Autodesk Inventor part; units mm, degrees
ref_plane "YZ Plane" through (0, 0, 0) normal (1, 0, 0) x (0, 1, 0)
ref_plane "XZ Plane" through (0, 0, 0) normal (0, 1, 0) x (-1, 0, 0)
ref_plane "XY Plane" through (0, 0, 0) normal (0, 0, 1) x (1, 0, 0)
sketch "Esboço1" plane through (0, 0, 0) normal (0, 0, 1) x (1, 0, 0)
  line L0 (0, 0) -> (-70, 0)
  line L1 (0, 0) -> (0, 30)
  line L2 (-70, 30) -> (-70, 28)
  line L3 (-70, 28) -> (-18, 28)
  line L4 (-18, 28) -> (-58.0179, 28)
  line L5 (-18, 28) -> (-18, 25)
  line L6 (-18, 25) -> (-6, 25)
  line L7 (-6, 25) -> (-6, 0)
  line L8 (0, 30) -> (-6, 30)
  line L9 (-6, 30) -> (-6, 27.5)
  line L10 (-6, 27.5) -> (-9, 27.5)
  line L11 (-9, 27.5) -> (-9, 30)
  line L12 (-9, 30) -> (-12, 30)
  line L13 (-12, 30) -> (-12, 27.5)
  line L14 (-12, 27.5) -> (-15, 27.5)
  line L15 (-15, 27.5) -> (-15, 30)
  line L16 (-15, 30) -> (-70, 30)
  line L17 (-6, 0) -> (0, 0)
  dimension "d1" = 60
  dimension "d2" = 70
  dimension "d4" = 70
  dimension "d5" = 56
  dimension "d8" = 52
  dimension "d9" = 64
  dimension "d10" = 50
  dimension "d11" = 6
  dimension "d12" = 55
  dimension "d13" = 3
  dimension "d14" = 3
  dimension "d15" = 3
  dimension "d16" = 55
  dimension "d17" = 55
  dimension "d18" = 60
revolve "Revolução1" add sketch "Esboço1" angle 360 about axis through (0, 0, 0) along (-1, 0, 0)
chamfer "Chanfro1" distance 2 angle 45 1 edges at (0, -30, 0)
fillet "Arredondamento1" radius 2 1 edges at (-18, -28, 0)
sketch "Esboço2" plane through (0, 0, 0) normal (0, 0, 1) x (1, 0, 0)
  line L0 (-70, 0) -> (-40, 0)
  line L1 (-70, 0) -> (-90, 0)
  circle A0 centre (-90, 0) radius 32.5
  point P0 (0, 0)
  dimension "d24" = 70
  dimension "d25" = 30
  dimension "d26" = 20
  dimension "d27" = 65
  dimension "d28" = 90
extrude "Extrusão1" cut sketch "Esboço2" along normal mid plane 200000
sketch "Esboço3" plane through (0, 0, 0) normal (0, 1, 0) x (-1, 0, 0)
  line L0 (70, -15.6125) -> (70, 15.6125)
  line L1 (70, 0) -> (40, 0)
  line L2 (70, -15.6125) -> (70, 15.6125)
  circle A0 centre (40, 0) radius 12.5
  point P0 (0, 0)
  dimension "d32" = 30
  dimension "d33" = 25
extrude "Extrusão2" add sketch "Esboço3" along normal up to next
sketch "Esboço4" plane through (-40, 0, 0) normal (0, -1, 0) x (1, 0, 0)
  circle A0 centre (0, 0) radius 12.5
  point P0 (40, 0)
extrude "Extrusão3" add sketch "Esboço4" along normal up to next
sketch "Esboço5" plane through (-6, 0, 0) normal (-1, 0, 0) x (0, 0, 1)
  line L0 (-17.5, -10) -> (17.5, -10)
  line L1 (17.5, -10) -> (17.5, 10)
  line L2 (17.5, 10) -> (-17.5, 10)
  line L3 (-17.5, 10) -> (-17.5, -10)
  line L4 (-17.5, -10) -> (17.5, 10) construction
  line L5 (17.5, -10) -> (-17.5, 10) construction
  point P0 (0, 0)
  dimension "d38" = 20
extrude "Extrusão4" cut sketch "Esboço5" along normal blind 100
sketch "Esboço6" plane through (-40, 10, 0) normal (0, -1, 0) x (1, 0, 0)
  circle A0 centre (0, 0) radius 12.5
  circle A1 centre (0, 0) radius 9
  point P0 (40, 0)
  dimension "d41" = 18
extrude "Extrusão5" cut sketch "Esboço6" along normal mid plane 100 contours A1
sketch "Esboço8" plane through (0, 0, 0) normal (0, 0, 1) x (1, 0, 0)
  line L0 (0, 0) -> (-31, 0)
  line L1 (-31, 27) -> (-29, 27)
  line L2 (-29, 27) -> (-29, 25)
  line L3 (-29, 25) -> (-31, 25)
  line L4 (-31, 27) -> (-31, 25)
  line L5 (-31, -27) -> (-29, -27)
  line L6 (-29, -27) -> (-29, -25)
  line L7 (-29, -25) -> (-31, -25)
  line L8 (-31, -27) -> (-31, -25)
  line L9 (-49, 30) -> (-49, 10)
  line L10 (-40, 30) -> (-40, -34.5055)
  point P0 (-31, 30)
  dimension "d45" = 3
  dimension "d46" = 2
  dimension "d47" = 2
  dimension "d49" = 18
revolve "Revolução2" cut sketch "Esboço8" angle 360 about axis through (-40, 30, 0) along (0, -1, 0)
properties part number "02"
Model file for the job. Use its own axes, mm. A direction names the side the tool comes from. Give positions to 0.01 mm unless a question says otherwise; leave off trailing zeros. Put each result on its own line as item: value. Start each with the question number.
(1) Tool access for faces 1 (the face through (-37, 10, 9)), 2 (the face through (-57.5, -0.1, -28.2)), 3 (the face through (-12, 13.2, 24.3)): list every direction of +Z, -Z, +X, -X, +Y, -Y with a clear straight run to the whole face (end or side of a thin tool).
(2) Band-saw the part on C-C on y = -23. Count the separate pieces of the cut face and the enclosed holes in it, then the cut area to 3 significant figures.
(3) Pin check, flat tips, straight feed: pin 1 Ø6 at (x, z) = (-22.5, -15) entering from +Y; pin 2 Ø6 at (x, z) = (-61, -6) entering from +Y; pin 3 Ø1.5 at (x, y) = (-57, 9.5) entering from -Z. Stop position of each tip, or through.
(4) Drill centre lines: L1, parallel to Z at x = -46.5, y = 0; L2, parallel to Z at x = -44, y = -16; L3, parallel to Z at x = -40, y = 15. Where is each one in solid material? Low to high. Write a range as [from, to].
(5) Pull direction Y, two halves, no side cores. Call faces 4 (the face through (-0.13, -6.1, 27.46)), 5 (the face through (-49, 17, 0)), 6 (the face through (-37.29, 18.874, 12.203)), 7 (the face through (-38, -25, -9)): released by +Y, released by -Y, zero draft, split by the parting line, or undercut.
Results below:
1. face 1: -X
1. face 2: +Z, -Z, -X
1. face 3: none
2. separate pieces: 2
2. enclosed holes: 1
2. area: 964 mm2
3. pin 1: stops at y = 27.5
3. pin 2: stops at y = 29.85
3. pin 3: stops at z = -28.7
4. L1: z = [-30, -28], [28, 30]
4. L2: z = [-25.38, -22.98], [-11.84, -8.06], [8.06, 11.84], [22.98, 25.38]
4. L3: z = [-25.98, -23.64], [-12.5, -9], [9, 12.5], [23.64, 25.98]
5. face 4: split by the parting line
5. face 5: zero draft
5. face 6: undercut
5. face 7: undercut
